Job drawing, mm, ordinate dimensions from the low corner. One solid piece. Give positions to 0.01 mm unless a question says otherwise; leave off trailing zeros. Loops run counter-clockwise (first coordinate to the right, second up) from the corner with the lowest first, then second, coordinate; pieces in that order, holes last. Notation, with made-up numbers: M 15.25,68.25 L 59.25,68.25 A21 cw 59.25,84.25 Z; hole C -32,-3.5 d2. An arc over 180 degrees is marked long. Answer in a Markdown table with one row per item.
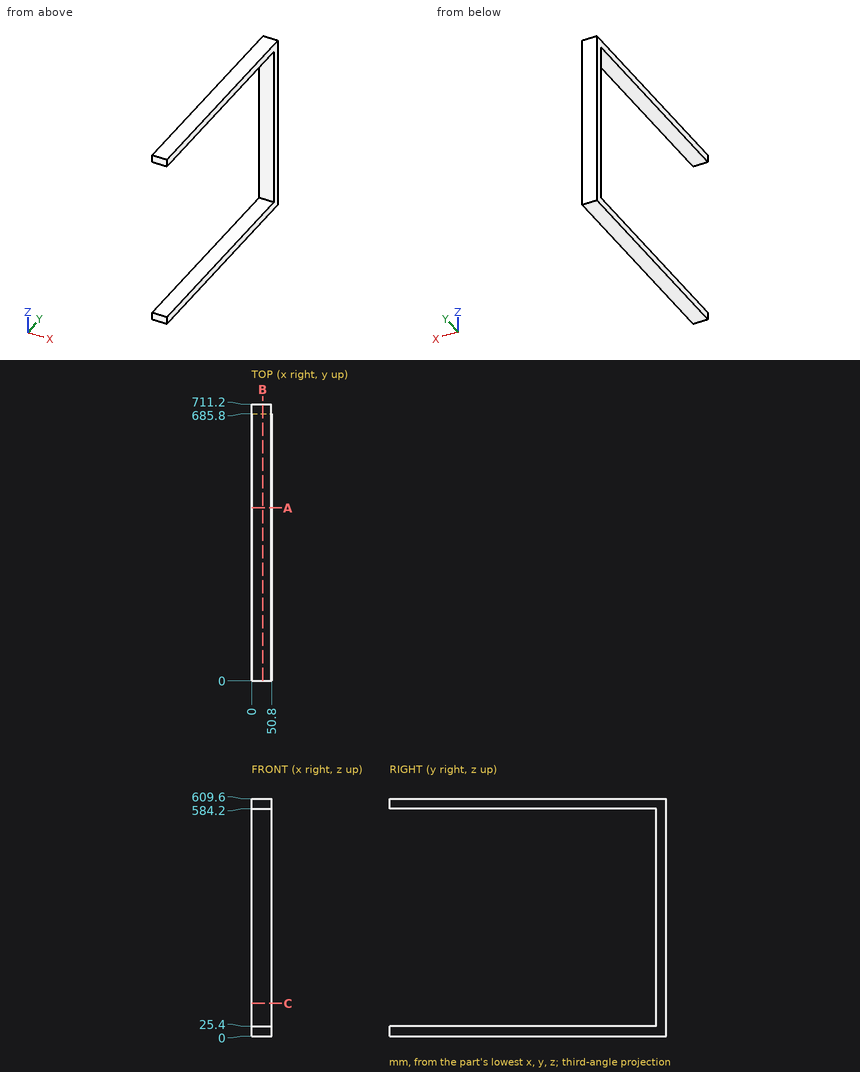
(1) Drill centre lines: line 1 along Z through (x, y) = (44, 591.5); line 2 along Y through (x, z) = (16, 234.5). Where is each one in solid material? Low to high.
Recorded:
| item | result |
|---|---|
| line 1 | z = 0 to 25.4, 584.2 to 609.6 |
| line 2 | y = 685.8 to 711.2 |
(2) Saw through at A-A (y = 444). Write the cut outline in (x, z), plus the area to 3 significant figures.
Recorded:
| item | result |
|---|---|
| outline | M 0,0 L 50.8,0 L 50.8,25.4 L 0,25.4 Z; M 0,584.2 L 50.8,584.2 L 50.8,609.6 L 0,609.6 Z |
| area | 2,580 mm^2 |
(3) Pin check, flat tip, straight feed: pin 1 Ø8 at (x, z) = (11.5, 154.5) entering from -Y. Stop position of the tip, or through.
Recorded:
| item | result |
|---|---|
| pin 1 | stops at y = 685.8 |
(4) Saw through at B-B (x = 28). Write the cut outline in (y, z).
Recorded:
| item | result |
|---|---|
| outline | M 0,0 L 711.2,0 L 711.2,609.6 L 0,609.6 L 0,584.2 L 685.8,584.2 L 685.8,25.4 L 0,25.4 Z |
(5) Saw through at C-C (z = 84). Write the cut outline in (x, y), plus the area to 3 significant figures.
Recorded:
| item | result |
|---|---|
| outline | M 0,685.8 L 50.8,685.8 L 50.8,711.2 L 0,711.2 Z |
| area | 1,290 mm^2 |
